from build123d import *

# Parameters (mm, degrees)
F0_W     = 25.4
F0_H     = 31.75
F1_DEPTH = 31.75
F2_W     = 6.35
F2_H     = 31.75
F3_DEPTH = 25.4
F4_W     = 25.4
F4_H     = 6.3268248923
F5_DEPTH = 25.4


with BuildPart() as f1:
    # F0 (on Right) → F1 (new body)
    with BuildSketch(Plane.YZ):
        with Locations((12.7, 15.875)):
            Rectangle(F0_W, F0_H)
    extrude(amount=F1_DEPTH)

    # F2 (on face) → F3 (join)
    with BuildSketch(Plane(origin=(0, 25.4, 0), x_dir=(-1, 0, 0), z_dir=(0, 1, 0))):
        with Locations((-3.175, 15.875)):
            Rectangle(F2_W, F2_H)
    extrude(amount=F3_DEPTH)

    # F4 (on face) → F5 (join)
    with BuildSketch(Plane.YZ.offset(6.35)):
        with Locations((38.1, 3.1634124462)):
            Rectangle(F4_W, F4_H)
    extrude(amount=F5_DEPTH)


solid = f1.part
Geometry: final body of the model. Coordinates: model frame, mm. A direction names the side the tool comes from. Coordinates: 2 decimals unless noted, no trailing zeros. Loops run counter-clockwise (first coordinate to the right, second up) from the corner with the lowest first, then second, coordinate; pieces in that order, holes last. Notation, with made-up numbers: M 20.25,68.25 L 45.25,68.25 A20 ccw 45.25,93.25 Z; hole C 31,-27.75 d3. An arc over 180 degrees is marked long. One line per item, written item: value. Start each with the question number.
1) Draft query along Y for faces 1 (the flat face through (16, 0, 16)), 2 (the flat face through (5, 50.8, 9)), 3 (the flat face through (0, 25, 16)). Return one class per face: released by +Y, released by -Y, zero draft, split by the parting line, or undercut.
2) Material intervals for L1, parallel to Y at x = 23.5, z = 17.5; L2, parallel to X at y = 39, z = 21; L3, parallel to Z at x = 12, y = 40.5, sorted ascending. Write a range as from..to.
3) Cut plane B-B (x = 9). Return loops of the section in (y, z).
4) Cut plane A-A (y = 47). Return loops of the section in (x, z).
5) Reachability of faces 4 (the flat face through (31.75, 19, 13)), 5 (the flat face through (6.35, 38, 19)) from +Z, -Z, +X, -X, +Y, -Y: full face, straight path, thin tool, end or side. Return the list, or none.
6) Pin query (flat end, axial travel): P1, Ø12.5, axis at x = 20, y = 37.5, coming from the +Z side; P2, Ø5, axis at x = 25, z = 15, coming from the +Y side; P3, Ø3, axis at y = 44, z = 10.5, coming from the +X side. Return the tip coordinate at first contact, or that it passes through.
Evaluation:
1. face 1: released by -Y
1. face 2: released by +Y
1. face 3: zero draft
2. L1: 0..25.4
2. L2: 0..6.35
2. L3: 0..6.33
3. outline: M 0,0 L 50.8,0 L 50.8,6.33 L 25.4,6.33 L 25.4,31.75 L 0,31.75 Z
4. outline: M 0,0 L 31.75,0 L 31.75,6.33 L 6.35,6.33 L 6.35,31.75 L 0,31.75 Z
5. face 4: +Z, -Z, +X, +Y, -Y
5. face 5: +Z, +X, +Y
6. P1: z = 6.33
6. P2: y = 25.4
6. P3: x = 6.35
